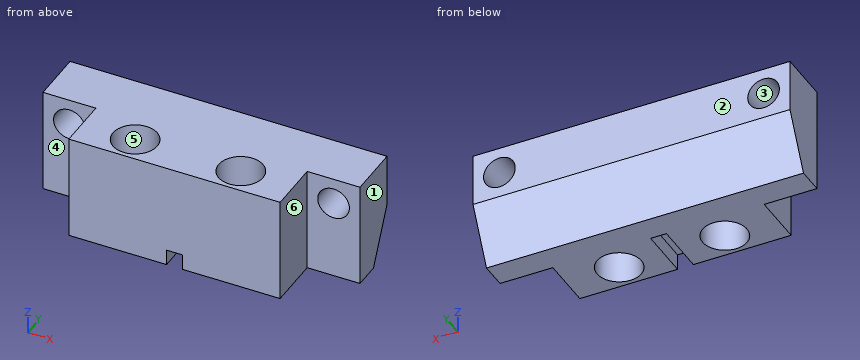
```python
from build123d import *

# Parameters (mm, degrees)
SKETCH1_W           = 30
SKETCH1_H           = 10
BOSS_EXTRUDE1_DEPTH = 5
SKETCH2_W           = 20
SKETCH2_H           = 10
BOSS_EXTRUDE2_DEPTH = 5
SKETCH3_R           = 2.1
CUT_EXTRUDE1_DEPTH  = 10
LPATTERN1_COUNT     = 2
LPATTERN1_PITCH     = 10
SKETCH4_R           = 1.5
CUT_EXTRUDE2_DEPTH  = 5
LPATTERN2_COUNT     = 2
LPATTERN2_PITCH     = 25
SKETCH5_W           = 1.5
SKETCH5_H           = 1.5
CUT_EXTRUDE3_DEPTH  = 5
CHAMFER1_SIZE       = 2.5
CHAMFER1_SIZE2      = 5


with BuildPart() as part:
    # Sketch1 → Boss-Extrude1 (new body)
    with BuildSketch(Plane(origin=(0, 0, 0), x_dir=(1, 0, 0), z_dir=(0, 1, 0))):
        with Locations((15, 5)):
            Rectangle(SKETCH1_W, SKETCH1_H)
    extrude(amount=BOSS_EXTRUDE1_DEPTH)

    # Sketch2 → Boss-Extrude2 (add)
    with BuildSketch(Plane.XZ):
        with Locations((15, -5)):
            Rectangle(SKETCH2_W, SKETCH2_H)
    extrude(amount=BOSS_EXTRUDE2_DEPTH)

    # Sketch3 → Cut-Extrude1 (cut)
    with BuildSketch(Plane.XY):
        with Locations((20, -2.5)):
            Circle(SKETCH3_R)
    cut_extrude1 = extrude(amount=-CUT_EXTRUDE1_DEPTH, mode=Mode.SUBTRACT)

    # LPattern1: Cut-Extrude1 ×2
    with Locations(*[(-i * LPATTERN1_PITCH, 0, 0) for i in range(1, LPATTERN1_COUNT)]):
        add(cut_extrude1, mode=Mode.SUBTRACT)

    # Sketch4 → Cut-Extrude2 (cut)
    with BuildSketch(Plane(origin=(0, 5, 0), x_dir=(1, 0, 0), z_dir=(0, 1, 0))):
        with Locations((27.5, 2.5)):
            Circle(SKETCH4_R)
    cut_extrude2 = extrude(amount=-CUT_EXTRUDE2_DEPTH, mode=Mode.SUBTRACT)

    # LPattern2: Cut-Extrude2 ×2
    with Locations(*[(-i * LPATTERN2_PITCH, 0, 0) for i in range(1, LPATTERN2_COUNT)]):
        add(cut_extrude2, mode=Mode.SUBTRACT)

    # Sketch5 → Cut-Extrude3 (cut)
    with BuildSketch(Plane.XZ.offset(5)):
        with Locations((15, -9.25)):
            Rectangle(SKETCH5_W, SKETCH5_H)
    extrude(amount=-CUT_EXTRUDE3_DEPTH, mode=Mode.SUBTRACT)

    # Chamfer1
    chamfer1_edges = [part.edges().sort_by_distance(p)[0] for p in [
        (15, 5, -10),
    ]]
    chamfer1_side = [part.faces().sort_by_distance(p)[0] for p in [
        (15, 0.991763931, -10),
    ]]
    chamfer(chamfer1_edges, length=CHAMFER1_SIZE, length2=CHAMFER1_SIZE2, reference=chamfer1_side[0])


solid = part.part
```
The model under review builds one solid part; all positions refer to its coordinate system, in mm. Face numbers are marked on the shaded views. A direction names the side the tool comes from. Round coordinates to 2 decimals unless told otherwise and drop trailing zeros. Write each loop counter-clockwise with the first axis right and the second up, starting at its lowest first coordinate (ties: lowest second). Pieces come first, ordered by that corner, then holes. Notation, with made-up numbers: M 73,79.25 L 97,79.25 A32 cw 97,105.25 Z; hole C -34,-9 d6. An arc over 180 degrees is marked long. Use CSV: the item, a comma, the result in double quotes. Start each with the question number.
(1) We need section B-B, the plane x = 2.5. State the section outline as (y, z) points, then the cut area to 4 significant figures.
(2) We need section C-C, the plane z = -2.5. State the section outline as (x, y) points.
(3) Tool access review of the marked faces 4, 5 and 6: name each direction out of +Z, -Z, +X, -X, +Y, -Y from which nothing blocks a thin tool from reaching the whole face with its end or side.
(4) For line 1 along X through (y, z) = (-1, -5); line 2 along X through (y, z) = (-1.75, -4.25); line 3 along Y through (x, z) = (10, -4.25), list the stretches that pass through material, from the lowest coordinate up.
(5) Clearance check with flat-ended pins moving along their axes: P1, Ø0.8, axis at y = -1.5, z = -9.5, coming from the -X side; P2, Ø1.5, axis at x = 28, z = -4.5, coming from the -Y side; P3, Ø1.5, axis at y = -3.5, z = -7, coming from the +X side. State where each tip first meets the part, or that it passes through.
(6) We need section D-D, the plane y = 4.25. State the section outline as (x, z) points, then the cut area to 3 significant figures.
(7) The part is to be moulded in two halves that separate along X. For the marked faces 1, 2 and 3, say which applies: +X half, -X half, draft (parallel to the pull), parting line (faces both ways), or undercut.
(8) We need section A-A, the plane y = -2.5. State the section outline as (x, z) points.
Findings:
1,outline,"M 0,-10 L 2.5,-10 L 5,-5 L 5,-4 L 0,-4 Z; M 0,-1 L 5,-1 L 5,0 L 0,0 Z"
1,area,"28.75 mm^2"
2,outline,"M 0,0 L 1,0 L 1,5 L 0,5 Z; M 4,0 L 5,0 L 5,-5 L 25,-5 L 25,0 L 26,0 L 26,5 L 4,5 Z; M 29,0 L 30,0 L 30,5 L 29,5 Z; hole C 10,-2.5 d4.2; hole C 20,-2.5 d4.2"
3,face 4,"+Z, -Z, -X, -Y"
3,face 5,"+Z, -Z"
3,face 6,"+Z, -Z, +X, -Y"
4,line 1,"5 to 8.53, 11.47 to 18.53, 21.47 to 25"
4,line 2,"5 to 8.04, 11.96 to 18.04, 21.96 to 25"
4,line 3,"-5 to -4.6, -0.4 to 5"
5,P1,"x = 5"
5,P2,"y = 0"
5,P3,"x = 25"
6,outline,"M 0,-6.5 L 30,-6.5 L 30,0 L 0,0 Z; hole C 2.5,-2.5 d3; hole C 27.5,-2.5 d3"
6,area,"181 mm^2"
7,face 1,"+X half"
7,face 2,"draft"
7,face 3,"undercut"
8,outline,"M 5,-10 L 7.9,-10 L 7.9,0 L 5,0 Z; M 12.1,-10 L 14.25,-10 L 14.25,-8.5 L 15.75,-8.5 L 15.75,-10 L 17.9,-10 L 17.9,0 L 12.1,0 Z; M 22.1,-10 L 25,-10 L 25,0 L 22.1,0 Z"
